Part model, mm, in its own coordinate system. A direction names the side the tool comes from. Round coordinates to 2 decimals unless told otherwise and drop trailing zeros. Loops run counter-clockwise (first coordinate to the right, second up) from the corner with the lowest first, then second, coordinate; pieces in that order, holes last.
1) Drop flat-ended pins along their axis: P1, Ø1.5, axis at y = 3.5, z = 2, coming from the +X side; P2, Ø0.9, axis at x = -3, y = 5.5, coming from the +Z side; P3, Ø0.6, axis at x = -2.5, z = -3, coming from the +Y side. Give the stop position or say it passes through.
2) Band-saw the part on A-A, the plane z = 0. Write the cut outline in (x, y), then the cut area to 3 significant figures.
3) Probe line 1 (Z direction, x = -2.95, y = 5.6); line 2 (Y direction, x = 2, z = -0.75); line 3 (X direction, y = 5.75, z = 1.25). List the from-to ranges inside material, lowest first.
4) Band-saw the part on B-B, the plane x = 0.75. Write the cut outline in (y, z).
5) 3-axis set-ups, long thin cutter, end or side, ignore diameter. For faces 4 (the flat face through (-1.3, -0.3, -3.25)), 5 (the flat face through (0, 0, -1)): which of +Z, -Z, +X, -X, +Y, -Y reach the whole face in a straight line?
6) Mould opens along Y. For faces 1 (the flat face through (-2.9, 8.7, -2)), 2 (the cylindrical face through (-2.86, 4.6, 0.32)), 3 (the flat face through (-1.3, -0.3, 3.25)) say: +Y half, -Y half, draft (parallel to the pull), parting line (faces both ways), or undercut.
7) Band-saw the part on D-D, the plane x = 2.5. Write the cut outline in (y, z), then the cut area to 3 significant figures.
8) Band-saw the part on C-C, the plane z = -2. Write the cut outline in (x, y), then the cut area to 3 significant figures.
from build123d import *

# Parameters (mm, degrees)
BASE_FLANGE1_DEPTH           = 0.8
EDGE_FLANGE1_STRIP_W         = 4.6732
EDGE_FLANGE1_STRIP_H         = 0.8
EDGE_FLANGE1_STRIP_CUT_DEPTH = 6.5
EDGE_FLANGE1_DEPTH           = 6.5
SKETCH10_W                   = 0.75
SKETCH10_H                   = 6.8
SKETCH10_R                   = 1.05
CUT_EXTRUDE1_DEPTH           = 12.724013818
BREAK_CORNER1_START          = 7.566042559
BREAK_CORNER1_OUTLINE_W      = 4
BREAK_CORNER1_OUTLINE_H      = 4.566042559
BREAK_CORNER1_DEPTH          = 0.707106781
BREAK_CORNER1_START_2        = 4.030508653
BREAK_CORNER1_2_OUTLINE_W    = 4
BREAK_CORNER1_2_OUTLINE_H    = 1.433957441
BREAK_CORNER1_2_DEPTH        = 1.414213562
SKETCH11_R                   = 1.05
CUT_EXTRUDE2_DEPTH           = 11.2842112


# Read off the part's stored shape, not the designer's step: Break-Corner1
# Sheet-metal steps are written as plain solids
with BuildPart() as part:
    # Sketch1 → Base-Flange1 (new body)
    with BuildSketch(Plane(origin=(0, 0, 0), x_dir=(1, 0, 0), z_dir=(0, 1, 0))):
        Polygon((1.75, 3.25), (3.25, 1.75), (3.25, -1.75), (1.75, -3.25), (-3.25, -3.25), (-3.25, 3.25), align=None)
    extrude(amount=-BASE_FLANGE1_DEPTH)

    # Edge-Flange1 strip (across the edge) → Edge-Flange1 strip cut (cut)
    with BuildSketch(Plane(origin=(-3.25, 0, -3.25), x_dir=(1, 0, 0), z_dir=(0, 0, 1))):
        with Locations((-0.8, -0.4)):
            Rectangle(EDGE_FLANGE1_STRIP_W, EDGE_FLANGE1_STRIP_H)
    extrude(amount=EDGE_FLANGE1_STRIP_CUT_DEPTH, mode=Mode.SUBTRACT)

    # Edge-Flange1 section (across the edge) → Edge-Flange1 (add)
    with BuildSketch(Plane(origin=(-3.25, 0, -3.25), x_dir=(1, 0, 0), z_dir=(0, 0, 1))):
        with BuildLine():
            Line((0, 0.7366), (0, 9.2))
            Line((0, 9.2), (0.8, 9.2))
            Line((0.8, 9.2), (0.8, 0.7366))
            ThreePointArc((0.8, 0.7366), (1.015745145, 0.215745145), (1.5366, 0))
            Line((1.5366, 0), (1.5366, -0.8))
            ThreePointArc((1.5366, -0.8), (0.45005972, -0.34994028), (0, 0.7366))
        make_face()
    extrude(amount=EDGE_FLANGE1_DEPTH)

    # Sketch10 → Cut-Extrude1 (cut, through all)
    with BuildSketch(Plane.ZY.offset(3.25)):
        with Locations((-2.875, 5.8)):
            Rectangle(SKETCH10_W, SKETCH10_H)
        with Locations((2.875, 5.8)):
            Rectangle(SKETCH10_W, SKETCH10_H)
        with Locations(Location((0, 5.6, 0), (0, 0, 270))):
            Circle(SKETCH10_R)
    extrude(amount=-CUT_EXTRUDE1_DEPTH, mode=Mode.SUBTRACT)

    # Break-Corner1 outline → Break-Corner1 (cut)
    with BuildSketch(Plane(origin=(0, 0, 0), x_dir=(1, 0, 0), z_dir=(0, 0.707106781186547, -0.707106781186548)).offset(BREAK_CORNER1_START)):
        with Locations((-3, -5.283021279)):
            Rectangle(BREAK_CORNER1_OUTLINE_W, BREAK_CORNER1_OUTLINE_H)
    extrude(amount=BREAK_CORNER1_DEPTH, mode=Mode.SUBTRACT)

    # Break-Corner1 2 outline → Break-Corner1 2 (cut)
    with BuildSketch(Plane(origin=(0, 0, 0), x_dir=(1, 0, 0), z_dir=(0, 0.707106781186547, -0.707106781186548)).offset(BREAK_CORNER1_START_2)):
        with Locations((-3, -8.283021279)):
            Rectangle(BREAK_CORNER1_2_OUTLINE_W, BREAK_CORNER1_2_OUTLINE_H)
    extrude(amount=BREAK_CORNER1_2_DEPTH, mode=Mode.SUBTRACT)

    # Sketch11 → Cut-Extrude2 (cut, through all)
    with BuildSketch(Plane(origin=(0, 0, 0), x_dir=(1, 0, 0), z_dir=(0, 1, 0))):
        with Locations(Location((0.75, 0, 0), (0, 0, 270))):
            Circle(SKETCH11_R)
    extrude(amount=-CUT_EXTRUDE2_DEPTH, mode=Mode.SUBTRACT)


solid = part.part
Reported:
1. P1: stops at x = -2.45
1. P2: stops at z = 2.5
1. P3: stops at y = 2.4
2. outline: (-3.25, 0.74) arc R1.54 ccw to (-1.71, -0.8) - (-0.3, -0.8) - (-0.3, 0) - (-1.71, 0) arc R0.74 cw to (-2.45, 0.74) - (-2.45, 4.55) - (-3.25, 4.55) - close; (-3.25, 6.65) - (-2.45, 6.65) - (-2.45, 9.2) - (-3.25, 9.2) - close; (1.8, -0.8) - (3.25, -0.8) - (3.25, 0) - (1.8, 0) - close
2. area: 8.81 mm2
3. line 1: z = -2.5 to -1.05, 1.05 to 2.5
3. line 2: y = -0.8 to 0
3. line 3: x = -3.25 to -2.45
4. outline: (-0.8, -3.25) - (0, -3.25) - (0, -1.05) - (-0.8, -1.05) - close; (-0.8, 1.05) - (0, 1.05) - (0, 3.25) - (-0.8, 3.25) - close
5. face 4: -Z, +X, -X, +Y, -Y
5. face 5: +Z, -Z, +X, +Y
6. face 1: +Y half
6. face 2: undercut
6. face 3: draft
7. outline: (-0.8, -2.5) - (0, -2.5) - (0, 2.5) - (-0.8, 2.5) - close
7. area: 4.00 mm2
8. outline: (-3.25, 0.74) arc R1.54 ccw to (-1.71, -0.8) - (3, -0.8) - (3, 0) - (-1.71, 0) arc R0.74 cw to (-2.45, 0.74) - (-2.45, 8.7) - (-3.25, 8.7) - close
8. area: 11.6 mm2
